Here's the drawing with two shaded views (mm, measured from the low corner). I have some questions. A direction names the side the tool comes from. Round coordinates to 2 decimals unless told otherwise and drop trailing zeros. Loops run counter-clockwise (first coordinate to the right, second up) from the corner with the lowest first, then second, coordinate; pieces in that order, holes last.
(1) I want a section at A-A on z = 16. Write out the boundary of the cut face in (x, y).
(2) I want a section at D-D on y = 61. Write out the boundary of the cut face in (x, z), plus the area to 3 significant figures.
(3) I want a section at C-C on z = 3.5. Write out the boundary of the cut face in (x, y), plus the area to 3 significant figures.
(4) Will this pin go through, and if not, where does the flat tip stop? pin 1 Ø12 at (x, y) = (23, 48.5) entering from +Z.
(5) Which directions (+Z, -Z, +X, -X, +Y, -Y) give clear straight access to the entire face, cutting with the end or side of a thin tool? Please do the marked faces 4 and 5.
(6) I want a section at B-B on y = 47.5. Write out the boundary of the cut face in (x, z).
(7) If I drill on line 1 along Y through (x, z) = (77.5, 23.5); line 2 along X through (y, z) = (51, 14); line 3 along Z through (x, y) = (86, 43.5), over which ranges is the centre line in solid material (lowest first)?
(8) Thinking about a two-plate mould opening in Y: for the marked faces 1, 2 and 3, which applies, released by +Y, released by -Y, zero draft, split by the parting line, or undercut?
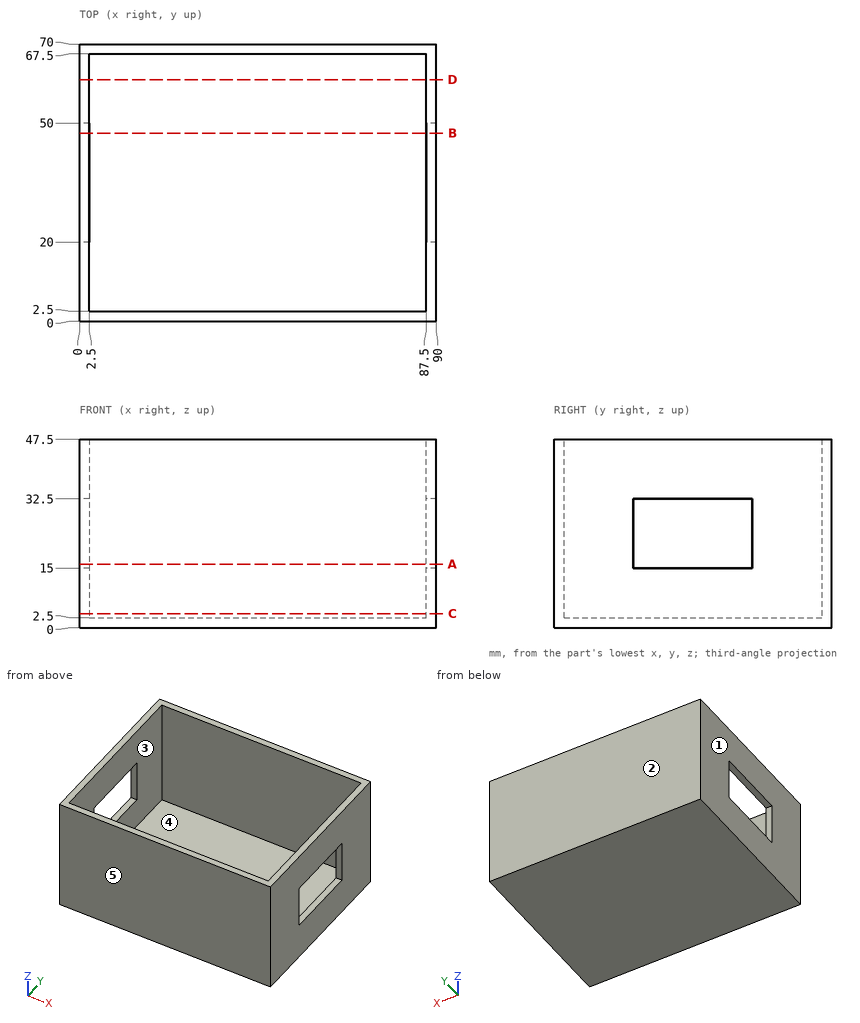
Filled sheet:
1. outline: (0, 0) - (90, 0) - (90, 20) - (87.5, 20) - (87.5, 2.5) - (2.5, 2.5) - (2.5, 20) - (0, 20) - close; (0, 50) - (2.5, 50) - (2.5, 67.5) - (87.5, 67.5) - (87.5, 50) - (90, 50) - (90, 70) - (0, 70) - close
2. outline: (0, 0) - (90, 0) - (90, 47.5) - (87.5, 47.5) - (87.5, 2.5) - (2.5, 2.5) - (2.5, 47.5) - (0, 47.5) - close
2. area: 450 mm2
3. outline: (0, 0) - (90, 0) - (90, 70) - (0, 70) - close; hole (2.5, 2.5) - (87.5, 2.5) - (87.5, 67.5) - (2.5, 67.5) - close
3. area: 775 mm2
4. pin 1: stops at z = 2.5
5. face 4: +Z
5. face 5: +Z, -Z, +X, -X, -Y
6. outline: (0, 0) - (90, 0) - (90, 15) - (87.5, 15) - (87.5, 2.5) - (2.5, 2.5) - (2.5, 15) - (0, 15) - close; (0, 32.5) - (2.5, 32.5) - (2.5, 47.5) - (0, 47.5) - close; (87.5, 32.5) - (90, 32.5) - (90, 47.5) - (87.5, 47.5) - close
7. line 1: y = 0 to 2.5, 67.5 to 70
7. line 2: x = 0 to 2.5, 87.5 to 90
7. line 3: z = 0 to 2.5
8. face 1: zero draft
8. face 2: released by +Y
8. face 3: undercut
